Build history of the part. All positions in model axes, mm. Give positions to 0.01 mm unless a question says otherwise; leave off trailing zeros. Order: outer loops, then holes, each group sorted by start corner. A loop starts at its lowest first (then second) coordinate and runs counter-clockwise, first axis right, second up. Notation, with made-up numbers: (-31, -32.75) - (-26, -32.75) arc R17 cw to (-26, -9.75) - close; hole circle Ø3 at (-25.75, -31). An arc over 180 degrees is marked (long way). Write each question's results on one line, items separated by ' | '. Start each with the question number.
1) Cut at D-D on x = -33.02. List the corners of the cut face in (y, z) (3 decimals), plus the area to 3 significant figures.
2) Cut at A-A on y = 25.4. List the corners of the cut face in (x, z).
3) Cut at B-B on x = 0. List the corners of the cut face in (y, z), plus the area to 3 significant figures.
4) Cut at C-C on z = 2.54. List the corners of the cut face in (x, y) (3 decimals).
5) Drop flat-ended pins along their axis: pin 1 Ø1.5 at (x, z) = (-18, 2.5) entering from -Y; pin 2 Ø3 at (x, z) = (-26.5, 1) entering from +Y; pin 3 Ø11.5 at (x, y) = (0, 0) entering from +Z. Give the stop position or say it passes through.
6) Drill centre lines: line 1 along Y through (x, z) = (0, 3.55); line 2 along Y through (x, z) = (-30, 4.35); line 3 along X through (y, z) = (-26.5, 4.65). Where is each one in solid material? Low to high. Write a range as from..to.
from build123d import *

# Parameters (mm, degrees)
F0_W     = 76.2
F0_H     = 76.2
F0_R     = 6.35
F1_DEPTH = 5.08
F2_R     = 1.905
F3_DEPTH = 5.08
F4_R     = 1.905
F5_DEPTH = 5.08


with BuildPart() as f1:
    # F0 (on Top) → F1 (new body)
    with BuildSketch(Plane.XY):
        Rectangle(F0_W, F0_H)
        with Locations((0, -25.4)):
            Circle(F0_R, mode=Mode.SUBTRACT)
        Circle(F0_R, mode=Mode.SUBTRACT)
        with Locations((0, 25.4)):
            Circle(F0_R, mode=Mode.SUBTRACT)
    extrude(amount=F1_DEPTH)

    # F2 (on face) → F3 (join)
    with BuildSketch(Plane.XZ.offset(38.1)):
        with Locations((-33.02, 2.54)):
            Circle(F2_R)
        with Locations((33.02, 2.54)):
            Circle(F2_R)
    extrude(amount=F3_DEPTH)

    # F4 (on face) → F5 (join)
    with BuildSketch(Plane(origin=(0, 38.1, 0), x_dir=(-1, 0, 0), z_dir=(0, 1, 0))):
        with Locations((-33.02, 2.54)):
            Circle(F4_R)
        with Locations((33.02, 2.54)):
            Circle(F4_R)
    extrude(amount=F5_DEPTH)


solid = f1.part
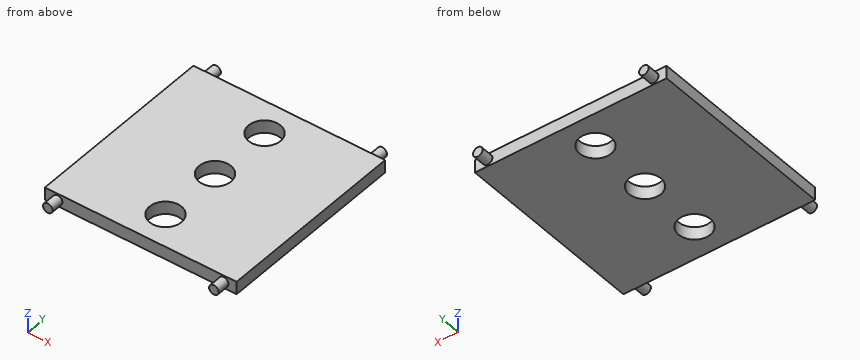
Results:
1) outline: (-43.18, 0.635) - (-38.1, 0.635) - (-38.1, 0) - (38.1, 0) - (38.1, 0.635) - (43.18, 0.635) - (43.18, 4.445) - (38.1, 4.445) - (38.1, 5.08) - (-38.1, 5.08) - (-38.1, 4.445) - (-43.18, 4.445) - close | area: 426 mm^2
2) outline: (-38.1, 0) - (-6.35, 0) - (-6.35, 5.08) - (-38.1, 5.08) - close; (6.35, 0) - (38.1, 0) - (38.1, 5.08) - (6.35, 5.08) - close
3) outline: (-38.1, 0) - (-31.75, 0) - (-31.75, 5.08) - (-38.1, 5.08) - close; (-19.05, 0) - (-6.35, 0) - (-6.35, 5.08) - (-19.05, 5.08) - close; (6.35, 0) - (19.05, 0) - (19.05, 5.08) - (6.35, 5.08) - close; (31.75, 0) - (38.1, 0) - (38.1, 5.08) - (31.75, 5.08) - close | area: 194 mm^2
4) outline: (-38.1, -38.1) - (-34.925, -38.1) - (-34.925, -43.18) - (-31.115, -43.18) - (-31.115, -38.1) - (31.115, -38.1) - (31.115, -43.18) - (34.925, -43.18) - (34.925, -38.1) - (38.1, -38.1) - (38.1, 38.1) - (34.925, 38.1) - (34.925, 43.18) - (31.115, 43.18) - (31.115, 38.1) - (-31.115, 38.1) - (-31.115, 43.18) - (-34.925, 43.18) - (-34.925, 38.1) - (-38.1, 38.1) - close; hole circle Ø12.7 at (0, -25.4); hole circle Ø12.7 at (0, 0); hole circle Ø12.7 at (0, 25.4)
5) pin 1: y = -38.1 | pin 2: y = 38.1 | pin 3: through
6) line 1: -38.1..-31.75, -19.05..-6.35, 6.35..19.05, 31.75..38.1 | line 2: -38.1..38.1 | line 3: -38.1..-6.25, 6.25..38.1
